Input: part model. Units: mm. Frame: model coordinates. A direction names the side the tool comes from. Give positions to 0.01 mm unless a question says otherwise; leave off trailing zeros. Loops run counter-clockwise (first coordinate to the right, second up) from the corner with the lowest first, then second, coordinate; pieces in that order, holes last. Notation, with made-up numbers: M 5,41.25 L 17,41.25 A18 cw 17,54.25 Z; hole C 85.5,48 d2. An arc over 180 degrees is marked long. One line per item, written item: value. Start each with the question number.
(1) Ray query, line 1 along Y through (x, z) = (0, 4.75) (1 decimal); line 2 along Y through (x, z) = (-0.5, 0.75); line 3 along Z through (x, y) = (13.5, 0). Return the intervals inside material, ascending. Write a range as from..to.
(2) Section A-A on x = 0. Output: boundary loops of the cut face in (y, z) (1 decimal), plus the area to 3 significant figures.
(3) Pin query (flat end, axial travel): P1, Ø7.5, axis at x = 0, y = 0, coming from the +Z side; P2, Ø4, axis at y = -8.5, z = 3, coming from the -X side; P3, Ø4, axis at x = -4.5, z = 7, coming from the +Y side. Return the tip coordinate at first contact, or that it passes through.
(4) Pull-direction query (Y, two-part tool) for faces 1 (the cylindrical face through (14.664, 6.08, 3.667)), 2 (the cylindrical face through (5.562, -0.079, 8.725)), 3 (the flat face through (10, 0, 6.35)); classes: released by +Y, released by -Y, zero draft, split by the parting line, or undercut.
(5) Section D-D on z = 1.5. Output: boundary loops of the cut face in (x, y) (3 decimals).
(6) Access query for faces 4 (the flat face through (1.2, -3.1, 7.823)), 5 (the flat face through (5, 3, 9.601)), 6 (the flat face through (-10, 0, 6.35)). Directions: +Z, -Z, +X, -X, +Y, -Y. A direction counts if a zero-diameter tool reaches every point of the face in a straight line with its end or side. Return the directions, or none.
(7) Section C-C on y = -12. Output: boundary loops of the cut face in (x, z) (3 decimals).
(8) Section B-B on y = 0. Output: boundary loops of the cut face in (x, z) (3 decimals), plus the area to 3 significant figures.
Autodesk Inventor part; units mm, degrees
ref_plane "YZ Plane" through (0, 0, 0) normal (1, 0, 0) x (0, 1, 0)
ref_plane "XZ Plane" through (0, 0, 0) normal (0, 1, 0) x (-1, 0, 0)
ref_plane "XY Plane" through (0, 0, 0) normal (0, 0, 1) x (1, 0, 0)
sketch "Sketch1" plane through (0, 0, 0) normal (0, 0, 1) x (1, 0, 0)
  circle A0 centre (0, 0) radius 15.875
  dimension "d0" = 31.75
extrude "Extrusion1" add sketch "Sketch1" along normal blind 6.35
sketch "Sketch2" plane through (0, 0, 0) normal (0, 1, 0) x (-1, 0, 0)
  line L0 (15.875, 6.35) -> (-15.875, 6.35)
  line L1 (0, 6.35) -> (-6.604, 6.35)
  line L2 (0, 6.35) -> (6.604, 6.35)
  line L3 (0, 9.6012) -> (-11.684, 9.6012)
  line L4 (0, 9.6012) -> (11.684, 9.6012)
  line L5 (11.684, 9.6012) -> (6.604, 6.35)
  line L6 (-6.604, 6.35) -> (-11.684, 9.6012)
  line L7 (0, 6.35) -> (0, 9.6012)
  point P0 (0, 0)
  dimension "d8" = 13.208
  dimension "d9" = 3.2512
  dimension "d10" = 23.368
  dimension "d29" = 11.684
  dimension "d30" = 6.604
extrude "Extrusion2" add sketch "Sketch2" along normal mid plane 31.75
sketch "Sketch3" plane through (-11.684, 15.875, 9.6012) normal (0, 0, 1) x (1, 0, 0)
  circle A0 centre (11.684, -15.875) radius 15.875
  line L0 (0, -31.75) -> (0, 0)
  circle A1 centre (11.684, -15.875) radius 19.7112
extrude "Extrusion3" cut sketch "Sketch3" against normal blind 3.2512 contours A0 L0 A1 | A0 L0 A1
sketch "Sketch4" plane through (0, 0, 6.35) normal (0, 0, 1) x (1, 0, 0)
  circle A0 centre (0, 0) radius 3.1623
  circle A1 centre (0, 9.4742) radius 3.1623
  circle A2 centre (0, -9.4742) radius 3.1623
  dimension "d15" = 6.3246
  dimension "d16" = 6.3246
  dimension "d17" = 6.3246
  dimension "d18" = 9.4742
  dimension "d19" = 9.4742
extrude "Extrusion4" cut sketch "Sketch4" along normal through all both and the other way through all
sketch "Sketch5" plane through (0, 0, 9.6012) normal (0, 0, 1) x (1, 0, 0)
  circle A0 centre (0, 9.4742) radius 3.1623
  arc A1 (2.9159, 4.7371) -> (-2.9159, 4.7371) centre (0, 9.4742) ccw
  circle A2 centre (0, -9.4742) radius 3.1623
  arc A3 (-2.9159, -4.7371) -> (2.9159, -4.7371) centre (0, -9.4742) ccw
  arc A4 (-2.9159, 4.7371) -> (-2.9159, -4.7371) centre (0, 0) ccw
  arc A5 (2.9159, -4.7371) -> (2.9159, 4.7371) centre (0, 0) ccw
  dimension "d23" = 11.1252
  dimension "d24" = 11.1252
extrude "Extrusion5" cut sketch "Sketch5" against normal blind 1.778
properties part number "hockey puck"
Output values:
1. line 1: y = -15.9..-12.6, -6.3..-3.2, 3.2..6.3, 12.6..15.9
1. line 2: y = -15.87..-12.6, -6.35..-3.12, 3.12..6.35, 12.6..15.87
1. line 3: z = 0..6.35
2. outline: M -15.9,0 L -12.6,0 L -12.6,7.8 L -15,7.8 L -15,9.6 L -15.9,9.6 Z; M -6.3,0 L -3.2,0 L -3.2,7.8 L -6.3,7.8 Z; M 3.2,0 L 6.3,0 L 6.3,7.8 L 3.2,7.8 Z; M 12.6,0 L 15.9,0 L 15.9,9.6 L 15,9.6 L 15,7.8 L 12.6,7.8 Z
2. area: 103 mm²
3. P1: stops at z = 7.82
3. P2: stops at x = -14.48
3. P3: stops at y = 15.68
4. face 1: split by the parting line
4. face 2: undercut
4. face 3: zero draft
5. outline: C 0,0 d31.75; hole C 0,-9.474 d6.325; hole C 0,0 d6.325; hole C 0,9.474 d6.325
6. face 4: +Z
6. face 5: +Z, +X, -X, +Y, -Y
6. face 6: -X, +Y, -Y
7. outline: M -10.393,0 L -1.903,0 L -1.903,7.823 L -4.956,7.823 L -4.956,9.601 L -10.393,9.601 L -10.393,8.775 L -6.604,6.35 L -10.393,6.35 Z; M 1.903,0 L 10.393,0 L 10.393,6.35 L 6.604,6.35 L 10.393,8.775 L 10.393,9.601 L 4.956,9.601 L 4.956,7.823 L 1.903,7.823 Z
8. outline: M -15.875,0 L -3.162,0 L -3.162,7.823 L -5.563,7.823 L -5.563,9.601 L -11.684,9.601 L -6.604,6.35 L -15.875,6.35 Z; M 3.162,0 L 15.875,0 L 15.875,6.35 L 6.604,6.35 L 11.684,9.601 L 5.563,9.601 L 5.563,7.823 L 3.162,7.823 Z
8. area: 192 mm²
